Autodesk Inventor part; units mm, degrees
ref_plane "YZ Plane" through (0, 0, 0) normal (1, 0, 0) x (0, 1, 0)
ref_plane "XZ Plane" through (0, 0, 0) normal (0, 1, 0) x (-1, 0, 0)
ref_plane "XY Plane" through (0, 0, 0) normal (0, 0, 1) x (1, 0, 0)
sketch "Sketch1" plane through (0, 0, 0) normal (0, 1, 0) x (-1, 0, 0)
  arc A0 (11.078, -10.268) -> (11.078, 14.332) centre (6.1141, 2.032) ccw
  line L0 (12.8056, -21.6164) -> (10.5439, 25.4442)
  line L1 (11.078, 14.332) -> (2.478, 14.332)
  line L2 (11.078, -10.268) -> (2.478, -10.268)
  line L3 (2.478, 14.332) -> (-4.322, 11.532)
  line L4 (2.478, -10.268) -> (-4.322, -7.468)
  line L5 (-4.322, 11.532) -> (-11.422, 8.832)
  line L6 (-4.322, -7.468) -> (-11.422, -4.768)
  arc A1 (-11.422, 8.832) -> (-11.422, -4.768) centre (-0.862, 2.032) ccw
  line L7 (22.1018, 19.039) -> (-15.8982, 19.039)
  line L8 (-15.8982, 19.039) -> (-15.8982, -14.961)
  line L9 (-15.8982, -14.961) -> (22.1018, -14.961)
  line L10 (22.1018, -14.961) -> (22.1018, 19.039)
  point P0 (0, 0)
  point P1 (11.078, 2.032)
  point P2 (19.378, 2.032)
  point P3 (12.8056, -21.6164)
  point P4 (10.5439, 25.4442)
  point P5 (-13.422, 2.032)
  dimension "d0" = 0
  dimension "d1" = 0
  dimension "d2" = 7.7
  dimension "d3" = 8.6
  dimension "d4" = 8.6
  dimension "d5" = 2.8
  dimension "d6" = 2.8
  dimension "d7" = 6.8
  dimension "d8" = 6.8
  dimension "d9" = 24.6
  dimension "d10" = 7.1
  dimension "d11" = 7.1
  dimension "d12" = 2.7
  dimension "d13" = 2.7
  dimension "d14" = 2
  dimension "d56" = 34
  dimension "d57" = 38
  dimension "d66" = 32.8
  dimension "d67" = 24.6
extrude "Extrusion1" add sketch "Sketch1" along normal blind 104.4 contours A0 L0 L9 L8 L7 L1 L3 L5 A1 L6 L4 L2 | A0 L0 L7 L10 L9
sketch "Sketch3" plane through (0, 104.4, 0) normal (0, 1, 0) x (1, 0, 0)
  line L0 (-11.078, -12.582) -> (-2.5615, -12.582)
  line L1 (-2.5615, -12.582) -> (3.6938, -10.0063)
  line L2 (4.322, -11.532) -> (-2.478, -14.332)
  line L3 (3.6938, -10.0063) -> (10.43, -7.2326)
  line L4 (10.43, 3.38) -> (-3.0811, 8.518)
  line L5 (-3.0811, 8.518) -> (-11.078, 8.518)
  arc A0 (-11.078, 8.518) -> (-11.078, -12.582) centre (-5.8566, -2.032) ccw
  arc A1 (10.43, -7.2326) -> (10.43, 3.38) centre (0.611, -1.9263) ccw
  line L6 (-2.478, -14.332) -> (-11.078, -14.332)
  line L7 (-11.078, 10.268) -> (-2.478, 10.268)
  line L8 (4.322, 7.468) -> (11.422, 4.768)
  arc A2 (11.422, -8.832) -> (11.422, 4.768) centre (0.862, -2.032) ccw
  arc A3 (-11.078, 10.268) -> (-11.078, -14.332) centre (-6.1141, -2.032) ccw
  line L9 (-19.5547, -18.0128) -> (14.794, -18.0128)
  line L10 (14.794, -18.0128) -> (14.794, 13.635)
  line L11 (14.794, 13.635) -> (-19.5547, 13.635)
  line L12 (-19.5547, 13.635) -> (-19.5547, -18.0128)
  point P0 (0, 0)
  point P1 (13.422, -2.032)
  point P2 (11.772, -1.9263)
  point P3 (-17.628, -2.032)
  point P4 (-19.378, -2.032)
  dimension "d31" = 1.75
  dimension "d32" = 1.75
  dimension "d33" = 1.65
  dimension "d34" = 180
  dimension "d35" = 1.65
  dimension "d36" = 1.65
  dimension "d37" = 1.75
  dimension "d38" = 0
extrude "Extrusion2" add sketch "Sketch3" against normal blind 4
fillet "Fillet3" radius 1 22 edges at (-19.378, 0, 2.032) (-6.778, 0, -10.268) (-6.778, 0, 14.332) (0.922, 0, 12.932) (7.872, 0, 10.182) (13.422, 0, 2.032) (7.872, 0, -6.118) (0.922, 0, -8.868) (-17.628, 100.4, 2.032) (-7.0795, 100.4, -8.518) (3.6744, 100.4, -5.949) (11.772, 100.4, 1.9263) (-6.8197, 100.4, 12.582) (3.9342, 100.4, 9.9073) (-11.078, 50.2, 14.332) (-2.478, 50.2, 14.332) (4.322, 50.2, 11.532) (11.422, 50.2, 8.832) (11.422, 50.2, -4.768) (4.322, 50.2, -7.468) (-2.478, 50.2, -10.268) (-11.078, 50.2, -10.268)
fillet "Fillet6" radius 10 4 edges at (-22.1018, 52.2, 19.039) (-22.1018, 52.2, -14.961) (15.8982, 52.2, -14.961) (15.8982, 52.2, 19.039)
sketch "Sketch5" plane through (15.8982, 1, 19.039) normal (1, 0, 0) x (0, 0, -1)
  line L0 (39, 35.2) -> (-4, 35.2)
  line L1 (-4, 35.2) -> (-4, 14.7)
  line L2 (-4, 14.7) -> (39, 14.7)
  line L3 (39, 14.7) -> (39, 35.2)
  line L4 (34, 0) -> (34, 102.4)
  line L5 (33, 103.4) -> (1, 103.4)
  point P0 (19.039, -1)
  dimension "d58" = 20.5
  dimension "d59" = 5
  dimension "d60" = 43
  dimension "d61" = 88.7
sketch "Sketch7" plane through (-22.1018, 1, -14.961) normal (-1, 0, 0) x (0, 0, 1)
  line L0 (37.3481, 2.34) -> (-4.8767, 2.34)
  line L1 (-4.8767, 2.34) -> (-4.8767, 7.45)
  line L2 (-4.8767, 7.45) -> (37.3481, 7.45)
  line L3 (37.3481, 7.45) -> (37.3481, 2.34)
  line L4 (1, -1) -> (33, -1)
  point P0 (14.961, -1)
  dimension "d72" = 3.34
  dimension "d73" = 5.11
sketch "Sketch9" plane through (15.8982, 103.4, -14.961) normal (0, 0, -1) x (-1, 0, 0)
  line L0 (37.5, -100.06) -> (38, -100.06)
  line L1 (37.5, -100.06) -> (27.5, -100.06)
  line L2 (27.5, -100.06) -> (27.5, -94.95)
  line L3 (27.5, -94.95) -> (37.5, -94.95)
  line L4 (37.5, -94.95) -> (37.5, -100.06)
  line L5 (37.5, -94.95) -> (38, -94.95)
  point P0 (15.8982, -103.4)
  point P1 (37.75, -94.95)
  dimension "d79" = 0
  dimension "d80" = 10
properties part number "PipetteSleeve_3DPrint"
Can you work these out from the model? Positions are in its coordinate system, mm. A direction names the side the tool comes from. Coordinates: 2 decimals unless noted, no trailing zeros. Order: outer loops, then holes, each group sorted by start corner. A loop starts at its lowest first (then second) coordinate and runs counter-clockwise, first axis right, second up.
1. I'm going to push a flat-ended pin straight in: pin 1 (8 mm diameter, centred on x = -18, y = 61, fed in from -Z). Where does the tip first touch, or does it pass through?
2. Thinking about a two-plate mould opening in X: for faces 1 (the face through (11.77, 102.92, 2)), 2 (the face through (6, 104.4, 10)), 3 (the face through (13, 53, -12)), which applies, +X half, -X half, draft (parallel to the pull), parting line (faces both ways), or undercut?
3. I need wall thicknesses on line 1 (Z direction, x = -9, y = 85); line 2 (Z direction, x = 4, y = 74.5); line 3 (X direction, y = 88.5, z = -2). Which ranges of each line are inside material? Lowest first, please.
4. If we section it at B-B (y = 52): Please give me the cut outline in (x, z).
5. For faces 4 (the face through (3.8, 102.9, -5.9)), 5 (the face through (3.767, 100.685, -6.236)), 6 (the face through (15.898, 51, 2)), which set-ups out of +Z, -Z, +X, -X, +Y, -Y let a thin tool reach every point of the face, with its end or its side?
6. If we section it at A-A (x = -9): Please give me the cut outline in (y, z), then the cut area to 4 significant figures.
7. If we section it at C-C (z = 16.5): Please give me the cut outline in (x, y), then the cut area to 3 significant figures.
Entries:
1. pin 1: stops at z = -14.78
2. face 1: undercut
2. face 2: draft
2. face 3: +X half
3. line 1: z = -14.96 to -10.27, 14.33 to 19.04
3. line 2: z = -14.96 to -7.6, 11.66 to 19.04
3. line 3: x = -22.1 to -18.75, 12.76 to 15.9
4. outline: (-22.1, -4.96) arc R10 ccw to (-12.1, -14.96) - (5.9, -14.96) arc R10 ccw to (15.9, -4.96) - (15.9, 9.04) arc R10 ccw to (5.9, 19.04) - (-12.1, 19.04) arc R10 ccw to (-22.1, 9.04) - close; hole (-11.27, -10.19) arc R1 ccw to (-10.88, -10.27) - (-2.68, -10.27) arc R1 ccw to (-2.3, -10.19) - (4.32, -7.47) - (11.11, -4.89) arc R1 ccw to (11.61, -4.47) arc R12.56 ccw to (11.61, 8.53) arc R1 ccw to (11.11, 8.95) - (4.32, 11.53) - (-2.3, 14.26) arc R1 ccw to (-2.68, 14.33) - (-10.88, 14.33) arc R1 ccw to (-11.27, 14.25) arc R13.26 ccw to start
5. face 4: +Y, -Y
5. face 5: -Y
5. face 6: +Z, -Z, +X, +Y, -Y
6. outline: (0, -14.96) - (104.4, -14.96) - (104.4, -8.52) - (101.4, -8.52) arc R1 ccw to (100.4, -9.52) - (100.4, -10.27) - (1, -10.27) arc R1 ccw to (0, -11.27) - close; (0, 15.33) arc R1 ccw to (1, 14.33) - (100.4, 14.33) - (100.4, 13.58) arc R1 ccw to (101.4, 12.58) - (104.4, 12.58) - (104.4, 19.04) - (0, 19.04) - close
6. area: 994.5 mm2
7. outline: (-18.76, 0) - (12.56, 0) - (12.56, 104.4) - (-18.76, 104.4) - close
7. area: 3,270 mm2
